Source: CAD feature listing. Evaluate the final solid. Frame: model axes, mm. Face numbers are marked on the shaded views. A direction names the side the tool comes from. Round coordinates to 2 decimals unless told otherwise and drop trailing zeros. Loops run counter-clockwise (first coordinate to the right, second up) from the corner with the lowest first, then second, coordinate; pieces in that order, holes last.
Item 1: Ray query, L1, parallel to X at y = 2.75, z = -5.5; L2, parallel to Z at x = 73.5, y = 7.75; L3, parallel to Z at x = -14, y = 7.5. Return the intervals inside material, ascending.
Item 2: Section query A-A on z = -3. Return loops of the section in (x, y), then the cut area to 3 significant figures.
Item 3: Access query for the marked faces 5 and 6. Directions: +Z, -Z, +X, -X, +Y, -Y. A direction counts if a zero-diameter tool reaches every point of the face in a straight line with its end or side. Return the directions, or none.
Item 4: First-contact query: P1, Ø1, axis at x = 18, y = 2.5, coming from the -Z side; P2, Ø3, axis at x = -71, y = 3, coming from the -Z side. Flat tips, straight axial feed; report the tip coordinate or a pass-through.
Item 5: Section query C-C on y = 4.25. Return loops of the section in (x, z).
Item 6: Pull-direction query (X, two-part tool) for the marked faces 1, 2, 3 and 4; classes: released by +X, released by -X, zero draft, split by the parting line, or undercut.
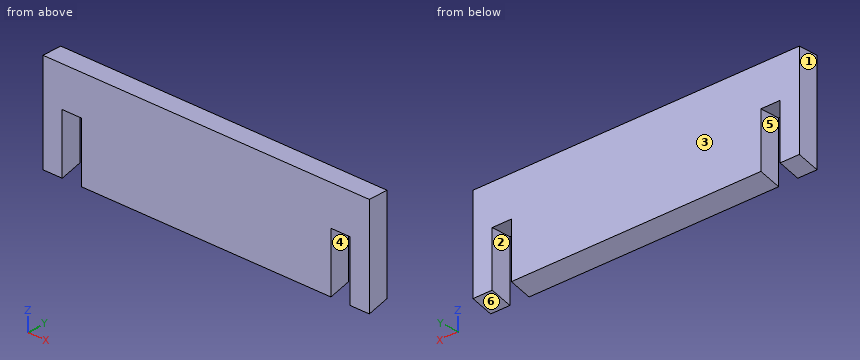
```python
from build123d import *

# Parameters (mm, degrees)
SKETCH2_W           = 170
SKETCH2_H           = 50
BOSS_EXTRUDE1_DEPTH = 10
CHAMFER1_SIZE2      = 2.679491924
CHAMFER1_SIZE       = 10
SKETCH4_W           = 10
SKETCH4_H           = 30
CUT_EXTRUDE1_DEPTH  = 10


with BuildPart() as part:
    # Sketch2 → Boss-Extrude1 (new body)
    with BuildSketch(Plane(origin=(0, 0, 0), x_dir=(1, 0, 0), z_dir=(0, 1, 0))):
        Rectangle(SKETCH2_W, SKETCH2_H)
    extrude(amount=BOSS_EXTRUDE1_DEPTH)

    # Chamfer1
    chamfer1_edges = [part.edges().sort_by_distance(p)[0] for p in [
        (0, 10, -25),
    ]]
    chamfer1_side = [part.faces().sort_by_distance(p)[0] for p in [
        (0, 9.946410162, -25),
    ]]
    chamfer(chamfer1_edges, length=CHAMFER1_SIZE - 0.0001, length2=CHAMFER1_SIZE2 - 0.0001, reference=chamfer1_side[0])  # a hair under: the kernel refuses the full size

    # Sketch4 → Cut-Extrude1 (cut)
    with BuildSketch(Plane(origin=(0, 0, 0), x_dir=(1, 0, 0), z_dir=(0, 1, 0))):
        with Locations((70, 10)):
            Rectangle(SKETCH4_W, SKETCH4_H)
        with Locations((-70, 10)):
            Rectangle(SKETCH4_W, SKETCH4_H)
    extrude(amount=CUT_EXTRUDE1_DEPTH, mode=Mode.SUBTRACT)


solid = part.part
```
Data:
1. L1: x = -85 to -75, -65 to 65, 75 to 85
1. L2: z = 5 to 25
1. L3: z = -22.99 to 25
2. outline: (-85, 0) - (-75, 0) - (-75, 10) - (-85, 10) - close; (-65, 0) - (65, 0) - (65, 10) - (-65, 10) - close; (75, 0) - (85, 0) - (85, 10) - (75, 10) - close
2. area: 1,500 mm2
3. face 5: -Z, +Y, -Y
3. face 6: -Z, +X, -X, +Y
4. P1: stops at z = -24.46
4. P2: stops at z = 5
5. outline: (-85, -23.86) - (-75, -23.86) - (-75, 5) - (-65, 5) - (-65, -23.86) - (65, -23.86) - (65, 5) - (75, 5) - (75, -23.86) - (85, -23.86) - (85, 25) - (-85, 25) - close
6. face 1: released by -X
6. face 2: undercut
6. face 3: zero draft
6. face 4: undercut
